Can you work these out from the drawing? Everything is in mm from the part's minimum corner. A direction names the side the tool comes from. Round coordinates to 2 decimals unless told otherwise and drop trailing zeros. Write each loop counter-clockwise with the first axis right and the second up, starting at its lowest first coordinate (ties: lowest second). Pieces come first, ordered by that corner, then holes. Notation, with made-up numbers: (48, -35) -> (95, -35) arc R15 ccw to (95, -20) -> close; hole circle Ø4 at (50, 55.5). An arc over 180 degrees is marked (long way). Write item = value, one per line. Start each with the question number.
1) I'm going to push flat-ended pins straight in: pin 1 (1.6 mm diameter, centred on x = 11.5, z = 8.5, fed in from -Y); pin 2 (6 mm diameter, centred on x = 30.5, z = 14.5, fed in from -Y); pin 3 (4 mm diameter, centred on x = 31, y = 18, fed in from +Z) (3 decimals). Where does each tip first touch, or does it pass through?
2) Imagine slicing it at D-D, the plane y = 4.25. Please give me the cut outline in (x, z) (3 decimals), then the cut area to 3 significant figures.
3) Imagine slicing it at C-C, the plane z = 9.5. Please give me the cut outline in (x, y) (3 decimals), then the cut area to 3 significant figures.
4) For the marked faces 5 and 6, which set-ups out of +Z, -Z, +X, -X, +Y, -Y let a thin tool reach every point of the face, with its end or its side?
5) Imagine slicing it at A-A, the plane y = 10.75. Please give me the cut outline in (x, z) (3 decimals).
6) Imagine slicing it at B-B, the plane x = 6. Please give me the cut outline in (y, z) (3 decimals), then the cut area to 3 significant figures.
7) If I drill on line 1 (X direction, y = 4, z = 10) (3 decimals); line 2 (X direction, y = 7.5, z = 16.25) (3 decimals); line 3 (Z direction, x = 22, y = 11.25) (3 decimals), over which ranges is the centre line in solid material (lowest first)?
8) Thinking about a two-plate mould opening in X: for the marked faces 1, 2, 3 and 4, which applies, +X half, -X half, draft (parallel to the pull), parting line (faces both ways), or undercut?
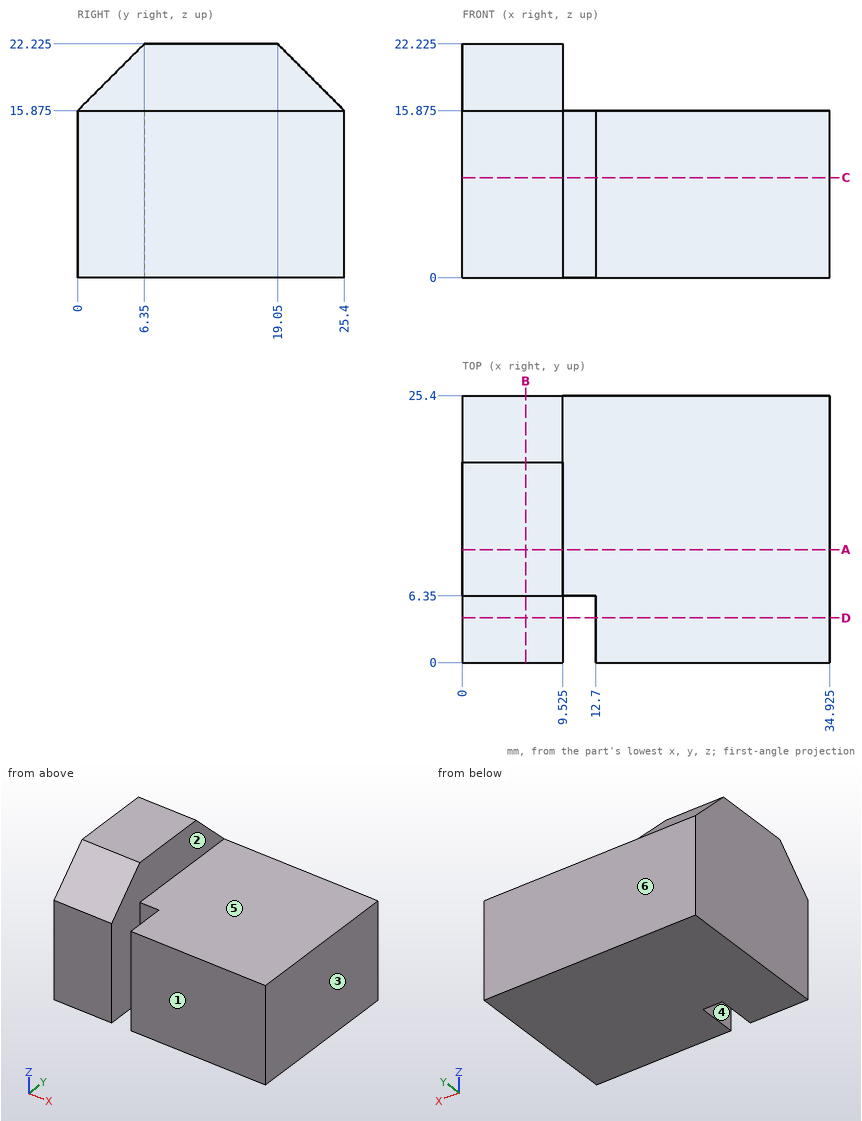
Reported:
q1.pin_1 = 6.35
q1.pin_2 = 0
q1.pin_3 = 15.875
q2.outline = (0, 0) -> (9.525, 0) -> (9.525, 20.125) -> (0, 20.125) -> close; (12.7, 0) -> (34.925, 0) -> (34.925, 15.875) -> (12.7, 15.875) -> close
q2.area = 545 mm²
q3.outline = (0, 0) -> (9.525, 0) -> (9.525, 6.35) -> (12.7, 6.35) -> (12.7, 0) -> (34.925, 0) -> (34.925, 25.4) -> (0, 25.4) -> close
q3.area = 867 mm²
q4.face_5 = +Z, +X, +Y, -Y
q4.face_6 = +Z, -Z, +X, -X, +Y
q5.outline = (0, 0) -> (34.925, 0) -> (34.925, 15.875) -> (9.525, 15.875) -> (9.525, 22.225) -> (0, 22.225) -> close
q6.outline = (0, 0) -> (25.4, 0) -> (25.4, 15.875) -> (19.05, 22.225) -> (6.35, 22.225) -> (0, 15.875) -> close
q6.area = 524 mm²
q7.line_1 = 0 to 9.525, 12.7 to 34.925
q7.line_2 = 0 to 9.525
q7.line_3 = 0 to 15.875
q8.face_1 = draft
q8.face_2 = undercut
q8.face_3 = +X half
q8.face_4 = undercut
